Geometry check sheet. Reference: drawing and pictorial views, mm from the part's lowest x, y, z. Give positions to 0.01 mm unless a question says otherwise; leave off trailing zeros. Loops run counter-clockwise (first coordinate to the right, second up) from the corner with the lowest first, then second, coordinate; pieces in that order, holes last. Notation, with made-up numbers: (67, -12) - (75, -12) arc R22 cw to (75, 16) - close; hole circle Ø9 at (86, -32.5). An arc over 180 degrees is marked (long way). Answer in a Markdown table with one row per item. Add a question column.
(1) Sectioned sample at B-B on x = 20. Enter the section's corners in (y, z).
(2) Go/stop test with flat-tipped pins: P1, Ø10, axis at x = 14.5, y = 26, coming from the -Z side; P2, Ø3, axis at x = 26.5, z = 12, coming from the +Y side; P3, Ø1.5, axis at y = 22, z = 20, coming from the -X side. Record where each tip stops, or that it passes through.
(3) Thickness scan on L1, parallel to X at y = 0.85, z = 19; L2, parallel to X at y = 4, z = 20; L3, parallel to Y at x = 36.5, z = 25. Record the ranges inside material, lowest first.
(4) Sectioned sample at A-A on z = 19. Enter the section's corners in (x, y), then the cut area to 3 significant figures.
(5) Sectioned sample at D-D on z = 25. Enter the section's corners in (x, y).
(6) Sectioned sample at C-C on y = 15. Enter the section's corners in (x, z), then the cut area to 3 significant figures.
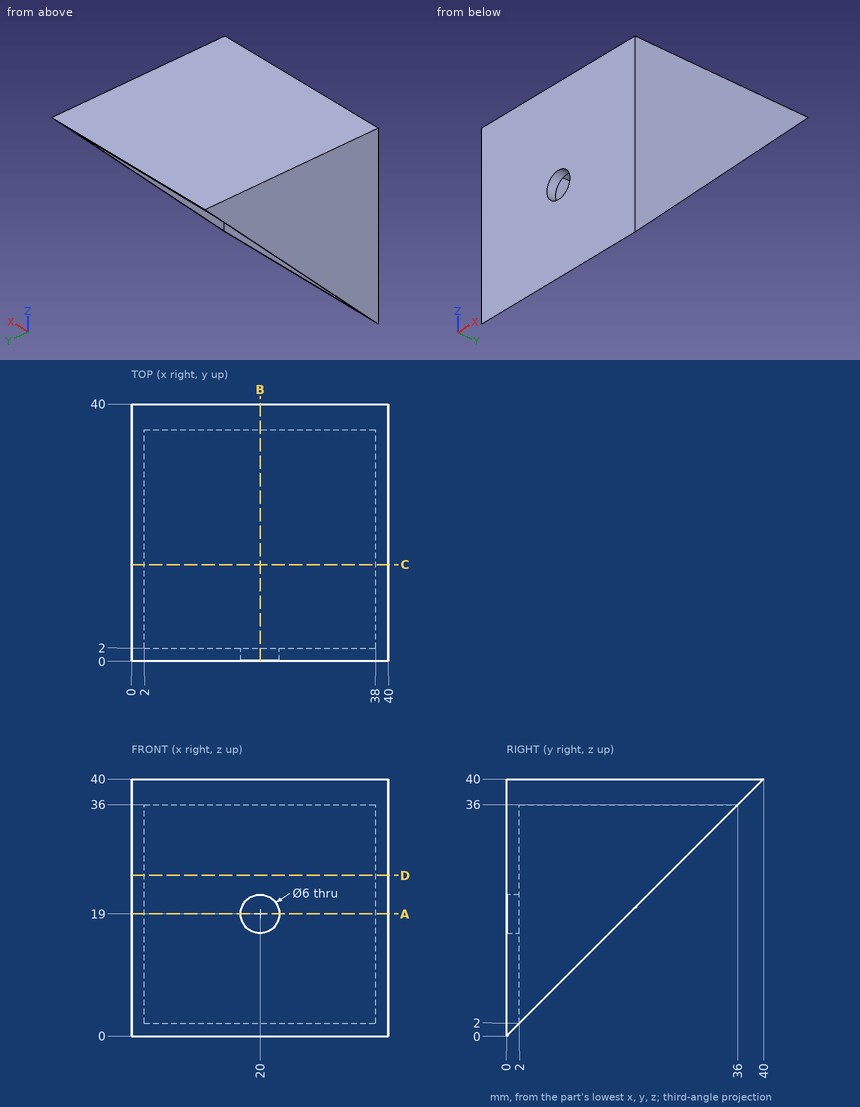
Reply:
| question | item | result |
|---|---|---|
| 1 | outline | (0, 0) - (2, 2) - (2, 16) - (0, 16) - close; (0, 22) - (2, 22) - (2, 36) - (36, 36) - (40, 40) - (0, 40) - close |
| 2 | P1 | z = 36 |
| 2 | P2 | y = 2 |
| 2 | P3 | through |
| 3 | L1 | 0 to 17, 23 to 40 |
| 3 | L2 | 0 to 2, 38 to 40 |
| 3 | L3 | 0 to 2 |
| 4 | outline | (0, 0) - (17, 0) - (17, 2) - (2, 2) - (2, 19) - (0, 19) - close; (23, 0) - (40, 0) - (40, 19) - (38, 19) - (38, 2) - (23, 2) - close |
| 4 | area | 136 mm^2 |
| 5 | outline | (0, 0) - (40, 0) - (40, 25) - (38, 25) - (38, 2) - (2, 2) - (2, 25) - (0, 25) - close |
| 6 | outline | (0, 15) - (2, 15) - (2, 36) - (38, 36) - (38, 15) - (40, 15) - (40, 40) - (0, 40) - close |
| 6 | area | 244 mm^2 |
